```python
from build123d import *

# Parameters (mm, degrees)
BOSS_EXTRUDE1_DEPTH     = 6.35
CUT_EXTRUDE1_DEPTH      = 57.9238307
CUT_EXTRUDE1_DEPTH_BACK = 57.9238307
SKETCH2_R               = 3.175


with BuildPart() as part:
    # Sketch1 → Boss-Extrude1 (new body)
    with BuildSketch(Plane.XY):
        with BuildLine():
            Line((5.674999953, 0), (40.00000001, 0))
            ThreePointArc((40.00000001, 0), (-28.284271255, -28.284271255), (0, 40.00000001))
            Line((0, 40.00000001), (0, 5.674999953))
            ThreePointArc((0, 5.674999953), (4.01283095, 4.01283095), (5.674999953, 0))
        make_face()
    extrude(amount=BOSS_EXTRUDE1_DEPTH)

    # Sketch2 → Cut-Extrude1 (cut, two sides: drawn at the far end of the back side and taken through both)
    with BuildSketch(Plane.XY.offset(6.35).offset(-CUT_EXTRUDE1_DEPTH_BACK)):
        Circle(SKETCH2_R)
    extrude(amount=CUT_EXTRUDE1_DEPTH + CUT_EXTRUDE1_DEPTH_BACK, mode=Mode.SUBTRACT)


solid = part.part
```
Can you work these out from the model? Positions are in its coordinate system, mm. A direction names the side the tool comes from. Round coordinates to 2 decimals unless told otherwise and drop trailing zeros. Order: outer loops, then holes, each group sorted by start corner. A loop starts at its lowest first (then second) coordinate and runs counter-clockwise, first axis right, second up.
(1) If we section it at A-A (z = 2): Please give me the cut outline in (x, y) (3 decimals).
Results are:
outline: (0, 5.675) - (0, 40) arc R40 ccw (long way) to (40, 0) - (5.675, 0) arc R5.675 ccw to start; hole circle Ø6.35 at (0, 0)
(2) If we section it at C-C (y = -27.5): Please give me the cut outline in (x, z).
Results are:
outline: (-29.05, 0) - (29.05, 0) - (29.05, 6.35) - (-29.05, 6.35) - close
(3) We'd pull the mould along X, two halves only. Please class faces 1 (the face through (-27.34, -29.2, 3.13)), 2 (the face through (-8, -8, 0)), 3 (the face through (3.968, 4.057, 3.131)), 4 (the face through (-0.69, -3.1, 3.13)): +X half, -X half, draft (parallel to the pull), parting line (faces both ways), or undercut.
Results are:
face 1: parting line
face 2: draft
face 3: +X half
face 4: undercut
(4) I'm going to push flat-ended pins straight in: pin 1 (2 mm diameter, centred on x = -7.5, z = 4.5, fed in from -Y); pin 2 (1.9 mm diameter, centred on y = 17, z = 1.5, fed in from +X); pin 3 (12 mm diameter, centred on x = 0, y = -2.5, fed in from -Z); pin 4 (1 mm diameter, centred on y = -17, z = 5.5, fed in from +X). Where does each tip first touch, or does it pass through?
Results are:
pin 1: stops at y = -39.47
pin 2: stops at x = 0
pin 3: stops at z = 0
pin 4: stops at x = 36.44
(5) On a 3-axis mill with a long thin cutter (end or side, diameter ignored), from which of +Z, -Z, +X, -X, +Y, -Y can I reach the whole of each face in a straight line? I mean faces 5 (the face through (0, 23, 3)), 6 (the face through (-8, -8, 6.35)). Say none if no direction works.
Results are:
face 5: +Z, -Z, +X, +Y
face 6: +Z, +X, -X, +Y, -Y
(6) If I drill on L1, parallel to X at y = -1, z = 4.5; L2, parallel to Y at x = 28.5, z = 4.25; L3, parallel to Y at x = -15, z = 4.75, over which ranges is the centre line in solid material (lowest first)?
Results are:
L1: x = -39.99 to -3.01, 3.01 to 39.99
L2: y = -28.07 to 0
L3: y = -37.08 to 37.08
(7) If we section it at B-B (x = 17): Please give me the cut outline in (y, z), plus the area to 3 significant figures.
Results are:
outline: (-36.21, 0) - (0, 0) - (0, 6.35) - (-36.21, 6.35) - close
area: 230 mm2
